The model under review builds one solid part; all positions refer to its coordinate system, in mm. A direction names the side the tool comes from. Round coordinates to 2 decimals unless told otherwise and drop trailing zeros. Loops run counter-clockwise (first coordinate to the right, second up) from the corner with the lowest first, then second, coordinate; pieces in that order, holes last. Notation, with made-up numbers: (55.25, 60.5) -> (75.25, 60.5) arc R19 ccw to (75.25, 71.5) -> close; hole circle Ø2 at (1.25, -7). An arc over 180 degrees is marked (long way). Return JSON: item names as keys, results as strings. Group by question number.
```python
from build123d import *

# Parameters (mm, degrees)
DODANIE_WYCI_GNI_CIE1_DEPTH = 12.5
SZKIC3_R                    = 13
WYTNIJ_WYCI_GNI_CIE1_DEPTH  = 7.5
SZKIC4_W                    = 7
SZKIC4_H                    = 35
DODANIE_WYCI_GNI_CIE2_DEPTH = 15
SZKIC6_R                    = 2
WYTNIJ_WYCI_GNI_CIE2_DEPTH  = 7
WYTNIJ_WYCI_GNI_CIE3_START  = -7
SZKIC7_R                    = 2
WYTNIJ_WYCI_GNI_CIE3_DEPTH  = 7
ZAOKR_GLENIE2_R             = 1.5
ZAOKR_GLENIE3_R             = 1.5
SZKIC8_W                    = 2.5
SZKIC8_H                    = 35
WYTNIJ_WYCI_GNI_CIE4_DEPTH  = 3.5
ZAOKR_GLENIE4_R             = 1


with BuildPart() as part:
    # Szkic2 → Dodanie-wyciągnięcie1 (new body)
    with BuildSketch(Plane.XY):
        with BuildLine():
            ThreePointArc((0, -10.5), (-10.5, 0), (0, 10.5))
            Line((0, 10.5), (-32, 10.5))
            Line((-32, 10.5), (-32, -10.5))
            Line((-32, -10.5), (0, -10.5))
        make_face()
        with BuildLine():
            Line((32, 10.5), (0, 10.5))
            ThreePointArc((0, 10.5), (7.424621202, 7.424621202), (10.5, 0))
            ThreePointArc((10.5, 0), (7.424621202, -7.424621202), (0, -10.5))
            Line((0, -10.5), (32, -10.5))
            Line((32, -10.5), (32, 10.5))
        make_face()
        Polygon((0, 10.5), (32, 10.5), (32, 17.5), (-32, 17.5), (-32, 10.5), align=None)
        Polygon((32, -10.5), (32, -17.5), (-32, -17.5), (-32, -10.5), (0, -10.5), align=None)
    extrude(amount=DODANIE_WYCI_GNI_CIE1_DEPTH)

    # Szkic3 → Wytnij-wyciągnięcie1 (cut)
    with BuildSketch(Plane.XY.offset(12.5)):
        Circle(SZKIC3_R)
    extrude(amount=-WYTNIJ_WYCI_GNI_CIE1_DEPTH, mode=Mode.SUBTRACT)

    # Szkic4 → Dodanie-wyciągnięcie2 (add)
    with BuildSketch(Plane.XY.offset(12.5)):
        with Locations((-28.5, 0)):
            Rectangle(SZKIC4_W, SZKIC4_H)
        with Locations((28.5, 0)):
            Rectangle(SZKIC4_W, SZKIC4_H)
    extrude(amount=DODANIE_WYCI_GNI_CIE2_DEPTH)

    # Szkic6 → Wytnij-wyciągnięcie2 (cut)
    with BuildSketch(Plane.ZY.offset(-25)):
        with Locations(Location((20, 0, 0), (0, 0, 270))):
            Circle(SZKIC6_R)
    extrude(amount=-WYTNIJ_WYCI_GNI_CIE2_DEPTH, mode=Mode.SUBTRACT)

    # Szkic7 → Wytnij-wyciągnięcie3 (cut)
    with BuildSketch(Plane(origin=(-25, 0, 0), x_dir=(0, 0, -1), z_dir=(1, 0, 0)).offset(WYTNIJ_WYCI_GNI_CIE3_START)):
        with Locations(Location((-20, 0, 0), (0, 0, 270))):
            Circle(SZKIC7_R)
    extrude(amount=WYTNIJ_WYCI_GNI_CIE3_DEPTH, mode=Mode.SUBTRACT)

    # Zaokrąglenie2
    zaokr_glenie2_edges = [part.edges().sort_by_distance(p)[0] for p in [
        (-13, 0, 12.5),
    ]]
    fillet(zaokr_glenie2_edges, radius=ZAOKR_GLENIE2_R)

    # Zaokrąglenie3
    zaokr_glenie3_edges = [part.edges().sort_by_distance(p)[0] for p in [
        (0, 10.5, 0),
    ]]
    fillet(zaokr_glenie3_edges, radius=ZAOKR_GLENIE3_R)

    # Szkic8 → Wytnij-wyciągnięcie4 (cut)
    with BuildSketch(Plane.XY.offset(27.5)):
        with Locations((-26.25, 0)):
            Rectangle(SZKIC8_W, SZKIC8_H)
        with Locations((26.25, 0)):
            Rectangle(SZKIC8_W, SZKIC8_H)
    extrude(amount=-WYTNIJ_WYCI_GNI_CIE4_DEPTH, mode=Mode.SUBTRACT)

    # Zaokrąglenie4
    zaokr_glenie4_edges = [part.edges().sort_by_distance(p)[0] for p in [
        (-25, 0, 24),
        (25, 0, 24),
    ]]
    fillet(zaokr_glenie4_edges, radius=ZAOKR_GLENIE4_R)


solid = part.part
```
1. We need section B-B, the plane z = 15. Write out the cut boundary in (x, y), then the cut area to 3 significant figures.
2. Wall thickness on line 1 (Y direction, x = -28, z = 20); line 2 (X direction, y = -8, z = 17); line 3 (Z direction, x = 30.75, y = 0): over which ranges is each line inside the solid? List them lowest first.
3. We need section D-D, the plane x = 24. Write out the cut boundary in (y, z).
4. For P1, Ø6.5, axis at y = 0, z = 20, coming from the -X side; P2, Ø1.5, axis at x = -2, z = 14.5, coming from the -Y side; P3, Ø17.5, axis at x = -8, y = -4, coming from the +Z side; P4, Ø6, axis at x = -7, y = 7.5, coming from the +Z side, all flat-tipped, find the tip position at first contact; note any pin that passes through.
5. We need section C-C, the plane z = 5.75. Write out the cut boundary in (x, y).
6. Draft analysis for pull direction Y (two halves, no side actions). For faces 1 (the face through (27.5, 0, 26)), 2 (the face through (-10.316, -7.91, 8.042)), 3 (the face through (0, 17.5, 7)), state which applies: pulls with the +Y half, pulls with the -Y half, needs draft (parallel to the pull), parting line crosses it, or undercut.
7. We need section A-A, the plane z = 20. Write out the cut boundary in (x, y), then the cut area to 3 significant figures.
8. Tool access review of faces 4 (the face through (-25, -0.2, 17.7)), 5 (the face through (-29, 0, 18)), 6 (the face through (-9, 6, 5)): name each direction out of +Z, -Z, +X, -X, +Y, -Y from which nothing blocks a thin tool from reaching the whole face with its end or side.
Check sheet entries:
{
 "1": {"outline": "(-32, -17.5) -> (-25, -17.5) -> (-25, 17.5) -> (-32, 17.5) -> close; (25, -17.5) -> (32, -17.5) -> (32, 17.5) -> (25, 17.5) -> close", "area": "490 mm²"},
 "2": {"line 1": "y = -17.5 to -2, 2 to 17.5", "line 2": "x = -32 to -25, 25 to 32", "line 3": "z = 0 to 18, 22 to 27.5"},
 "3": {"outline": "(-17.5, 0) -> (17.5, 0) -> (17.5, 12.5) -> (-17.5, 12.5) -> close"},
 "4": {"P1": "stops at x = -32", "P2": "passes through", "P3": "stops at z = 12.5", "P4": "stops at z = 11.84"},
 "5": {"outline": "(-32, -17.5) -> (32, -17.5) -> (32, 17.5) -> (-32, 17.5) -> close; hole circle Ø26 at (0, 0)"},
 "6": {"face 1": "needs draft", "face 2": "undercut", "face 3": "pulls with the +Y half"},
 "7": {"outline": "(-32, -17.5) -> (-25, -17.5) -> (-25, -2) -> (-32, -2) -> close; (-32, 2) -> (-25, 2) -> (-25, 17.5) -> (-32, 17.5) -> close; (25, -17.5) -> (32, -17.5) -> (32, -2) -> (25, -2) -> close; (25, 2) -> (32, 2) -> (32, 17.5) -> (25, 17.5) -> close", "area": "434 mm²"},
 "8": {"face 4": "+Z, +Y, -Y", "face 5": "+X, -X", "face 6": "+Z"}
}
